Autodesk Inventor part; units mm, degrees
ref_plane "YZ Plane" through (0, 0, 0) normal (1, 0, 0) x (0, 1, 0)
ref_plane "XZ Plane" through (0, 0, 0) normal (0, 1, 0) x (-1, 0, 0)
ref_plane "XY Plane" through (0, 0, 0) normal (0, 0, 1) x (1, 0, 0)
sketch "Sketch1" plane through (0, 0, 0) normal (0, 1, 0) x (-1, 0, 0)
  line L0 (9, 16.5) -> (-9, 16.5)
  line L1 (-9, 16.5) -> (-9, -16.5)
  line L2 (-9, -16.5) -> (9, -16.5)
  line L3 (9, -16.5) -> (9, 16.5)
  line L4 (9, 16.5) -> (-9, -16.5) construction
  line L5 (-9, 16.5) -> (9, -16.5) construction
  point P0 (0, 0)
  dimension "d0" = 18
  dimension "d1" = 33
extrude "Extrusion1" add sketch "Sketch1" along normal blind 1.5
sketch "Sketch2" plane through (0, 1.5, 0) normal (0, 1, 0) x (1, 0, 0)
  line L0 (-3.8, -18.95) -> (3.8, -18.95)
  line L1 (3.8, -18.95) -> (3.8, -14.05)
  line L2 (3.8, -14.05) -> (-3.8, -14.05)
  line L3 (-3.8, -14.05) -> (-3.8, -18.95)
  line L4 (-9, -16.5) -> (9, -16.5)
  line L5 (-3.8, -18.95) -> (3.8, -14.05) construction
  line L6 (3.8, -18.95) -> (-3.8, -14.05) construction
  point P0 (0, 0)
  point P1 (0, -16.5)
  dimension "d4" = 7.6
  dimension "d5" = 4.9
extrude "Extrusion2" add sketch "Sketch2" along normal blind 2.5
properties part number "microplaceholder" material "Aluminum 6061"
Input: part model. Units: mm. Frame: model coordinates. A direction names the side the tool comes from. Give positions to 0.01 mm unless a question says otherwise; leave off trailing zeros. Order: outer loops, then holes, each group sorted by start corner. A loop starts at its lowest first (then second) coordinate and runs counter-clockwise, first axis right, second up. Notation, with made-up numbers: (-30.5, 25) - (-1.5, 25) arc R29 ccw to (-1.5, 52) - close; hole circle Ø2 at (79, 25.5). An arc over 180 degrees is marked (long way). Answer as a JSON object with one key per item and string values. Group by question number.
Q1. Cut plane C-C, the plane y = 0.8. Output: boundary loops of the cut face in (x, z).
Q2. Cut plane B-B, the plane z = 17.5. Output: boundary loops of the cut face in (x, y).
Q3. First-contact query: pin 1 Ø0.8 at (x, y) = (2, 1) entering from +Z; pin 2 Ø1.2 at (y, z) = (2.5, 17.5) entering from +X; pin 3 Ø0.7 at (x, z) = (-1, 18) entering from -Y. Flat tips, straight axial feed; report the tip coordinate or a pass-through.
Q4. Cut plane A-A, the plane x = -1.75. Output: boundary loops of the cut face in (y, z).
Q5. Line query: probe 1 along Y at (x, z) = (-8, -14); probe 2 along Z at (x, y) = (0.75, 0.75); probe 3 along Z at (x, y) = (0.5, 3.3). Output: solid intervals per line, ascending.
Q6. Set-up query: faces 1 (the face through (0, 3, 14.05)), 2 (the face through (3.8, 3, 17)), 3 (the face through (0, 1, 16.5)). Return all of +Z, -Z, +X, -X, +Y, -Y with unobstructed straight access to the full face (end or side cutting, diameter ignored); none if empty.
Results:
{
 "1": {"outline": "(-9, -16.5) - (9, -16.5) - (9, 16.5) - (-9, 16.5) - close"},
 "2": {"outline": "(-3.8, 1.5) - (3.8, 1.5) - (3.8, 4) - (-3.8, 4) - close"},
 "3": {"pin 1": "z = 16.5", "pin 2": "x = 3.8", "pin 3": "y = 1.5"},
 "4": {"outline": "(0, -16.5) - (1.5, -16.5) - (1.5, 14.05) - (4, 14.05) - (4, 18.95) - (1.5, 18.95) - (1.5, 16.5) - (0, 16.5) - close"},
 "5": {"probe 1": "0 to 1.5", "probe 2": "-16.5 to 16.5", "probe 3": "14.05 to 18.95"},
 "6": {"face 1": "-Z, +X, -X, +Y", "face 2": "+Z, -Z, +X, +Y", "face 3": "+Z, +X, -X, -Y"}
}
